from build123d import *

# Parameters (mm, degrees)
SKETCH1_W              = 140
SKETCH1_H              = 80
SKETCH1_R              = 1.7
SKETCH1_R_2            = 1.85
SKETCH1_W_2            = 30
SKETCH1_H_2            = 64
BOSS_EXTRUDE1_DEPTH    = 3
LIPO_STRAP_DEPTH       = 3
FILLET1_R              = 3
WALL_DEPTH             = 30
WALL_DIRECTION_2_REACH = 88.341
SKETCH4_W              = 30
SKETCH4_H              = 6.07780277
SKETCH4_R              = 2.05
SERVO_BOLTS_DEPTH      = 4
SKETCH5_W              = 4
SKETCH5_H              = 74
LIPO_WALL_DEPTH        = 30
SKETCH6_R              = 3.5
SKETCH6_R_2            = 2
SKETCH6_R_3            = 2.75
PCB_STANDOFF_DEPTH     = 18
SKETCH8_W              = 4
SKETCH8_H              = 3
WIRE_2_DEPTH           = 12
SKETCH9_W              = 84.893473151
SKETCH9_H              = 106.193160462
CUT_EXTRUDE3_DEPTH     = 20
FILLET2_R              = 3
SKETCH10_W             = 46.265699575
SKETCH10_H             = 26
CUT_EXTRUDE4_DEPTH     = 1.6
SKETCH11_W             = 7.044911652
SKETCH11_H             = 1.491863032
SKETCH11_W_2           = 16
SKETCH11_H_2           = 1.5
BOSS_EXTRUDE6_DEPTH    = 18
FILLET4_R              = 3
FILLET5_R              = 2
FILLET6_R              = 3
SKETCH12_W             = 35
SKETCH12_H             = 100
CUT_EXTRUDE5_DEPTH     = 6
FILLET7_R              = 2
BOSS_EXTRUDE7_DEPTH    = 25
SKETCH14_W             = 20.051449776
SKETCH14_H             = 30
CUT_EXTRUDE6_DEPTH     = 18


with BuildPart() as part:
    # Sketch1 → Boss-Extrude1 (new body)
    with BuildSketch(Plane.XY):
        with Locations((-6.457193845, 0)):
            Rectangle(SKETCH1_W, SKETCH1_H)
        with Locations((-8.5, 34.8)):
            Circle(SKETCH1_R, mode=Mode.SUBTRACT)
        with Locations((8.5, 34.8)):
            Circle(SKETCH1_R, mode=Mode.SUBTRACT)
        with Locations(Location((8.5, -34.8, 0), (0, 0, 180))):
            Circle(SKETCH1_R, mode=Mode.SUBTRACT)
        with Locations(Location((-8.5, -34.8, 0), (0, 0, 180))):
            Circle(SKETCH1_R, mode=Mode.SUBTRACT)
        with Locations((-40, 18.5)):
            Circle(SKETCH1_R_2, mode=Mode.SUBTRACT)
        with Locations(Location((-40, -18.5, 0), (0, 0, 180))):
            Circle(SKETCH1_R_2, mode=Mode.SUBTRACT)
        Rectangle(SKETCH1_W_2, SKETCH1_H_2, mode=Mode.SUBTRACT)
        with BuildLine():
            Line((19.542806155, -11), (19.542806155, 11))
            ThreePointArc((19.542806155, 11), (21.542806155, 13), (23.542806155, 11))
            Line((23.542806155, 11), (23.542806155, -11))
            ThreePointArc((23.542806155, -11), (21.542806155, -13), (19.542806155, -11))
        make_face(mode=Mode.SUBTRACT)
    extrude(amount=BOSS_EXTRUDE1_DEPTH)

    # Sketch2 → lipo strap (cut)
    with BuildSketch(Plane.XY.offset(3)):
        with BuildLine():
            Line((61.042806155, -11), (61.042806155, 11))
            ThreePointArc((61.042806155, 11), (63.542806155, 13.5), (66.042806155, 11))
            Line((66.042806155, 11), (66.042806155, -11))
            ThreePointArc((66.042806155, -11), (63.542806155, -13.5), (61.042806155, -11))
        make_face()
    extrude(amount=-LIPO_STRAP_DEPTH, mode=Mode.SUBTRACT)

    # Fillet1
    fillet1_edges = [part.edges().sort_by_distance(p)[0] for p in [
        (63.542806155, -40, 1.5),
        (-76.457193845, -40, 1.5),
        (-76.457193845, 40, 1.5),
        (63.542806155, 40, 1.5),
    ]]
    fillet(fillet1_edges, radius=FILLET1_R)

    # Sketch3 → wall (add)
    with BuildSketch(Plane.XY.offset(3)):
        with BuildLine():
            Line((60.542806155, 13.5), (63.642806155, 13.5))
            Line((63.642806155, 13.5), (63.642806155, 37))
            ThreePointArc((63.642806155, 37), (62.734837176, 39.192031022), (60.542806155, 40.1))
            Line((60.542806155, 40.1), (-73.457193845, 40.1))
            ThreePointArc((-73.457193845, 40.1), (-75.649224867, 39.192031022), (-76.557193845, 37))
            Line((-76.557193845, 37), (-76.557193845, -37))
            ThreePointArc((-76.557193845, -37), (-75.649224867, -39.192031022), (-73.457193845, -40.1))
            Line((-73.457193845, -40.1), (60.542806155, -40.1))
            ThreePointArc((60.542806155, -40.1), (62.734837176, -39.192031022), (63.642806155, -37))
            Line((63.642806155, -37), (63.642806155, -13.5))
            Line((63.642806155, -13.5), (60.542806155, -13.5))
            Line((60.542806155, -13.5), (60.542806155, -34))
            ThreePointArc((60.542806155, -34), (59.664126498, -36.121320344), (57.542806155, -37))
            Line((57.542806155, -37), (-70.457193845, -37))
            ThreePointArc((-70.457193845, -37), (-72.578514189, -36.121320344), (-73.457193845, -34))
            Line((-73.457193845, -34), (-73.457193845, 34))
            ThreePointArc((-73.457193845, 34), (-72.578514189, 36.121320344), (-70.457193845, 37))
            Line((-70.457193845, 37), (57.542806155, 37))
            ThreePointArc((57.542806155, 37), (59.664126498, 36.121320344), (60.542806155, 34))
            Line((60.542806155, 34), (60.542806155, 13.5))
        make_face()
    extrude(amount=WALL_DEPTH)

    # wall direction 2: up to this face of the body (flat: up to its plane)
    wall_direction_2_end = Plane(part.part.faces().sort_by_distance((-74.844742296, 0, 0))[0])
    # Sketch3 → wall direction 2 (add, up to the picked face)
    with BuildSketch(Plane.XY.offset(3), mode=Mode.PRIVATE) as wall_direction_2_sk1:
        with BuildLine():
            Line((60.542806155, 13.5), (63.642806155, 13.5))
            Line((63.642806155, 13.5), (63.642806155, 37))
            ThreePointArc((63.642806155, 37), (62.734837176, 39.192031022), (60.542806155, 40.1))
            Line((60.542806155, 40.1), (-73.457193845, 40.1))
            ThreePointArc((-73.457193845, 40.1), (-75.649224867, 39.192031022), (-76.557193845, 37))
            Line((-76.557193845, 37), (-76.557193845, -37))
            ThreePointArc((-76.557193845, -37), (-75.649224867, -39.192031022), (-73.457193845, -40.1))
            Line((-73.457193845, -40.1), (60.542806155, -40.1))
            ThreePointArc((60.542806155, -40.1), (62.734837176, -39.192031022), (63.642806155, -37))
            Line((63.642806155, -37), (63.642806155, -13.5))
            Line((63.642806155, -13.5), (60.542806155, -13.5))
            Line((60.542806155, -13.5), (60.542806155, -34))
            ThreePointArc((60.542806155, -34), (59.664126498, -36.121320344), (57.542806155, -37))
            Line((57.542806155, -37), (-70.457193845, -37))
            ThreePointArc((-70.457193845, -37), (-72.578514189, -36.121320344), (-73.457193845, -34))
            Line((-73.457193845, -34), (-73.457193845, 34))
            ThreePointArc((-73.457193845, 34), (-72.578514189, 36.121320344), (-70.457193845, 37))
            Line((-70.457193845, 37), (57.542806155, 37))
            ThreePointArc((57.542806155, 37), (59.664126498, 36.121320344), (60.542806155, 34))
            Line((60.542806155, 34), (60.542806155, 13.5))
        make_face()
    wall_direction_2_tool1 = split(extrude(wall_direction_2_sk1.sketch, amount=-WALL_DIRECTION_2_REACH, mode=Mode.PRIVATE), bisect_by=wall_direction_2_end, keep=Keep.BOTH, mode=Mode.PRIVATE)
    add(wall_direction_2_tool1.solids().sort_by(Axis((62.157987, 23.75, 3), (0, 0, -1)))[0])

    # Sketch4 → servo bolts (add)
    # profile 1 of 2: a face of its own
    with BuildSketch(Plane.XY.offset(3)):
        with Locations((0, 35.038901385)):
            Rectangle(SKETCH4_W, SKETCH4_H)
        with Locations((-8.5, 34.8)):
            Circle(SKETCH4_R, mode=Mode.SUBTRACT)
        with Locations((8.5, 34.8)):
            Circle(SKETCH4_R, mode=Mode.SUBTRACT)
    # profile 2 of 2: a face of its own
    with BuildSketch(Plane.XY.offset(3)):
        with Locations((0, -35.038901385)):
            Rectangle(SKETCH4_W, SKETCH4_H)
        with Locations(Location((8.5, -34.8, 0), (0, 0, 180))):
            Circle(SKETCH4_R, mode=Mode.SUBTRACT)
        with Locations(Location((-8.5, -34.8, 0), (0, 0, 180))):
            Circle(SKETCH4_R, mode=Mode.SUBTRACT)
    extrude(amount=SERVO_BOLTS_DEPTH)

    # Sketch5 → lipo wall (add)
    with BuildSketch(Plane.XY.offset(3)):
        with Locations((17, 0)):
            Rectangle(SKETCH5_W, SKETCH5_H)
    extrude(amount=LIPO_WALL_DEPTH)

    # Sketch6 → PCB standoff (add)
    # profile 1 of 2: a face of its own
    with BuildSketch(Plane.XY.offset(3)):
        with Locations(Location((-40, 18.5, 0), (0, 0, 180))):
            Circle(SKETCH6_R)
        with Locations((-40, 18.5)):
            Circle(SKETCH6_R_2, mode=Mode.SUBTRACT)
    # profile 2 of 2: a face of its own
    with BuildSketch(Plane.XY.offset(3)):
        with Locations(Location((-40, -18.5, 0), (0, 0, 180))):
            Circle(SKETCH6_R_3)
        with Locations((-40, -18.5)):
            Circle(SKETCH6_R_2, mode=Mode.SUBTRACT)
    extrude(amount=PCB_STANDOFF_DEPTH)

    # Sketch8 → wire 2 (cut)
    with BuildSketch(Plane.XY.offset(33)):
        with Locations((17, 35.5)):
            Rectangle(SKETCH8_W, SKETCH8_H)
    extrude(amount=-WIRE_2_DEPTH, mode=Mode.SUBTRACT)

    # Sketch9 → Cut-Extrude3 (cut)
    with BuildSketch(Plane.XY.offset(33)):
        with Locations((61.446736576, 0)):
            Rectangle(SKETCH9_W, SKETCH9_H)
    extrude(amount=-CUT_EXTRUDE3_DEPTH, mode=Mode.SUBTRACT)

    # Fillet2
    fillet2_edges = [part.edges().sort_by_distance(p)[0] for p in [
        (60.542806155, -23.75, 3),
        (59.664126498, -36.121320344, 3),
        (60.542806155, 23.75, 3),
        (59.664126498, 36.121320344, 3),
        (15, -37, 20),
        (15, 37, 14),
        (38.271403077, -37, 3),
        (19, -37, 8),
        (38.271403077, 37, 3),
        (19, 37, 8),
    ]]
    fillet(fillet2_edges, radius=FILLET2_R)

    # Sketch10 → Cut-Extrude4 (cut)
    with BuildSketch(Plane(origin=(0, 0, 0), x_dir=(-1, 0, 0), z_dir=(0, 0, -1))):
        with Locations((-44.675655943, 0)):
            Rectangle(SKETCH10_W, SKETCH10_H)
    extrude(amount=-CUT_EXTRUDE4_DEPTH, mode=Mode.SUBTRACT)

    # Sketch11 → Boss-Extrude6 (add)
    with BuildSketch(Plane.XY.offset(3)):
        with Locations((-40, -21.25)):
            Rectangle(SKETCH11_W, SKETCH11_H)
        with Locations((-32, 21.25)):
            Rectangle(SKETCH11_W_2, SKETCH11_H_2)
    extrude(amount=BOSS_EXTRUDE6_DEPTH)

    # Fillet4
    # the kernel refuses this fillet: 3 mm, written as the material it adds along each edge
    with BuildSketch(Plane(origin=(-41.883138208, -20.504068484, 21), x_dir=(-1.0, 1.8919573654777327e-12, 0), z_dir=(0, 0, -1))) as fillet4_piece_1:
        with BuildLine():
            CenterArc((3.866859234, 2.009492063), FILLET4_R, 180.05404317, 41.999955364)
            ThreePointArc((0.866860568, 2.006662369), (0.641374229, 0.913501222), (0, 0))
            Line((0, 0), (1.639317618, 0))
        make_face()
    extrude(amount=18)
    with BuildSketch(Plane(origin=(-38.116861792, -20.504068484, 21), x_dir=(1.0, 1.887622984429e-12, 0), z_dir=(0, 0, -1))) as fillet4_piece_2:
        with BuildLine():
            CenterArc((3.866859234, -2.009492063), FILLET4_R, 137.946001469, 41.999955362)
            ThreePointArc((0.866860568, -2.006662369), (0.641374229, -0.913501222), (0, 0))
            Line((0, 0), (1.639317618, 0))
        make_face()
    extrude(amount=18)
    with BuildSketch(Plane(origin=(-37.127718677, 20.5, 21), x_dir=(1, 0, 0), z_dir=(0, 0, -1))) as fillet4_piece_3:
        with BuildLine():
            CenterArc((3.550334966, 3), FILLET4_R, 188.849883098, 81.150116902)
            ThreePointArc((0.586050525, 2.538461538), (0.538013756, 1.212670671), (0, 0))
            Line((0, 0), (3.550334966, 0))
        make_face()
    extrude(amount=18)

    # Fillet5
    fillet5_edges = [part.edges().sort_by_distance(p)[0] for p in [
        (-36.477544174, -21.25, 3),
        (-43.522455826, -21.25, 3),
        (-40, -21.995931516, 3),
        (-42.658440839, 16.223447275, 3),
        (-24, 21.25, 3),
        (-32, 22, 3),
        (-40, -15.75, 3),
        (-28.788691855, 20.5, 3),
        (-35.528714617, 19.778663576, 3),
        (-37.04972894, -19.572320447, 3),
        (-42.95027106, -19.572320447, 3),
    ]]
    fillet(fillet5_edges, radius=FILLET5_R)

    # Fillet6
    fillet6_edges = [part.edges().sort_by_distance(p)[0] for p in [
        (19, 40.1, 23),
        (19, -40.1, 23),
    ]]
    fillet(fillet6_edges, radius=FILLET6_R)

    # Sketch12 → Cut-Extrude5 (cut)
    with BuildSketch(Plane.XY.offset(13)):
        with Locations((41.292806155, 0)):
            Rectangle(SKETCH12_W, SKETCH12_H)
    extrude(amount=-CUT_EXTRUDE5_DEPTH, mode=Mode.SUBTRACT)

    # Fillet7
    fillet7_edges = [part.edges().sort_by_distance(p)[0] for p in [
        (58.792806155, 38.413589014, 7),
        (58.792806155, -38.413589014, 7),
        (23.792806155, -38.55, 7),
        (23.792806155, 38.55, 7),
    ]]
    fillet(fillet7_edges, radius=FILLET7_R)

    # Sketch13 → Boss-Extrude7 (add)
    with BuildSketch(Plane.XY.offset(3)):
        with BuildLine():
            Line((-70.957193845, 31.5), (-70.957193845, 0.014955839))
            Line((-70.957193845, 0.014955839), (-68.457193845, 0.014955839))
            Line((-68.457193845, 0.014955839), (-68.457193845, 29))
            ThreePointArc((-68.457193845, 29), (-67.578514189, 31.121320344), (-65.457193845, 32))
            Line((-65.457193845, 32), (-15, 32))
            Line((-15, 32), (-15, 34.5))
            Line((-15, 34.5), (-67.957193845, 34.5))
            ThreePointArc((-67.957193845, 34.5), (-70.078514189, 33.621320344), (-70.957193845, 31.5))
        make_face()
    extrude(amount=BOSS_EXTRUDE7_DEPTH)

    # Sketch14 → Cut-Extrude6 (cut)
    with BuildSketch(Plane.XY.offset(33)):
        with Locations((15, 0)):
            Rectangle(SKETCH14_W, SKETCH14_H)
    extrude(amount=-CUT_EXTRUDE6_DEPTH, mode=Mode.SUBTRACT)


solid = part.part
The model under review builds one solid part; all positions refer to its coordinate system, in mm. A direction names the side the tool comes from. Coordinates: 2 decimals unless noted, no trailing zeros. Loops run counter-clockwise (first coordinate to the right, second up) from the corner with the lowest first, then second, coordinate; pieces in that order, holes last.
(1) Consider section A-A, the plane x = 8.5. Give the boundary of the cut face in (y, z).
Determined:
outline: (-40.1, 0) - (-36.5, 0) - (-36.5, 3) - (-36.85, 3) - (-36.85, 7) - (-37, 7) - (-37, 33) - (-40.1, 33) - close; (-33.1, 0) - (-32, 0) - (-32, 7) - (-32.75, 7) - (-32.75, 3) - (-33.1, 3) - close; (32, 0) - (33.1, 0) - (33.1, 3) - (32.75, 3) - (32.75, 7) - (32, 7) - close; (36.5, 0) - (40.1, 0) - (40.1, 33) - (37, 33) - (37, 7) - (36.85, 7) - (36.85, 3) - (36.5, 3) - close
(2) Draft analysis for pull direction Y (two halves, no side actions). For faces 6 (the flat face through (41, -39, 7)), 7 (the cylindrical face through (-41.364, 19.75, 1.479)), state which applies: +Y half, -Y half, draft (parallel to the pull), parting line (faces both ways), or undercut.
Determined:
face 6: draft
face 7: undercut
(3) Tool access review of faces 1 (the flat face through (21, 38, 13)), 2 (the flat face through (21, -38, 13)), 3 (the cylindrical face through (-72.6, -36.1, 17.8)), 4 (the cylindrical face through (62.086, 13.032, 1.854)), 5 (the flat face through (62, 27, 13)): name each direction out of +Z, -Z, +X, -X, +Y, -Y from which nothing blocks a thin tool from reaching the whole face with its end or side.
Determined:
face 1: +Z, +X, +Y
face 2: +Z, +X, -Y
face 3: +Z
face 4: +Z, -Z, +X
face 5: +Z, +X, +Y, -Y
(4) Consider section D-D, the plane x = 36. Give the boundary of the cut face in (y, z), plus the area to 3 significant figures.
Determined:
outline: (-40.1, 0) - (-13, 0) - (-13, 1.6) - (13, 1.6) - (13, 0) - (40.1, 0) - (40.1, 7) - (37, 7) - (37, 6) arc R3 cw to (34, 3) - (-34, 3) arc R3 cw to (-37, 6) - (-37, 7) - (-40.1, 7) - close
area: 228 mm2
(5) Wall thickness on L1, parallel to X at y = -34.8, z = 0.7; L2, parallel to Y at x = 8.5, z = 0.7; L3, parallel to Y at x = -20.5, z = 24.5: over which ranges is each line inside the solid? List them lowest first.
Determined:
L1: x = -76.56 to -10.2, -6.8 to 6.8, 10.2 to 63.64
L2: y = -40.1 to -36.5, -33.1 to -32, 32 to 33.1, 36.5 to 40.1
L3: y = -40.1 to -37, 32 to 34.5, 37 to 40.1
(6) Insertion check: P1, Ø21, axis at x = 46.5, y = -5.5, coming from the -Z side; P2, Ø0.9, axis at y = -9, z = 1, coming from the +X side; P3, Ø2.5, axis at y = -1, z = 1, coming from the +X side; P4, Ø4, axis at y = 14.5, z = 16.5, coming from the +X side. Each pin has a flat end and moves straight along its axis. Give the tip position at first contact, or say it passes through.
Determined:
P1: stops at z = 0
P2: stops at x = 19.54
P3: stops at x = 61.04
P4: stops at x = 19
(7) Consider section C-C, the plane z = 17.5. Give the number of separate pieces and of enclosed holes in the cut face, plus the area to 3 significant figures.
Determined:
separate pieces: 4
enclosed holes: 2
area: 1,290 mm2
(8) Consider section B-B, the plane y = 9. Give the boundary of the cut face in (x, z), plus the area to 3 significant figures.
Determined:
outline: (-76.56, 0) - (-15, 0) - (-15, 3) - (-68.46, 3) - (-68.46, 28) - (-70.96, 28) - (-70.96, 3) - (-73.46, 3) - (-73.46, 33) - (-76.56, 33) - close; (15, 0) - (19.54, 0) - (19.54, 3) - (19, 3) - (19, 15) - (15, 15) - close; (23.54, 1.6) - (61.04, 1.6) - (61.04, 3) - (23.54, 3) - close
area: 454 mm2
